Source: CAD feature listing. Evaluate the final solid. Frame: model axes, mm. Give positions to 0.01 mm unless a question says otherwise; leave off trailing zeros. Write each loop counter-clockwise with the first axis right and the second up, starting at its lowest first coordinate (ties: lowest second). Pieces come first, ordered by that corner, then holes. Notation, with made-up numbers: (80, -30.75) -> (99, -30.75) arc R23 cw to (99, 1.25) -> close; hole circle Ø3 at (-24, 59.5). An arc over 180 degrees is marked (long way). Use one line per item in the form item = value. Start each with the question number.
(1) Cut plane B-B, the plane y = 1.9. Output: boundary loops of the cut face in (x, z).
(2) Cut plane C-C, the plane x = -4. Output: boundary loops of the cut face in (y, z), and give its area (3 significant figures).
(3) Cut plane D-D, the plane y = -1.8. Output: boundary loops of the cut face in (x, z), and give its area (3 significant figures).
(4) Cut plane A-A, the plane z = 15. Output: boundary loops of the cut face in (x, y), and give its area (3 significant figures).
(5) Material intervals for line 1 along Z through (x, y) = (-0.5, -2.15); line 2 along Z through (x, y) = (3.5, -1.65); line 3 along X through (y, z) = (2.3, -13.5), sorted ascending. Write a range as from..to.
from build123d import *

# Parameters (mm, degrees)
BOSS_EXTRUDE1_DEPTH = 17.5
CUT_EXTRUDE1_START  = -2.5
CUT_EXTRUDE1_DEPTH  = 5


# Read off the part's stored shape, not the designer's step: Cut-Extrude1
with BuildPart() as part:
    # Sketch1 → Boss-Extrude1 (new, symmetric)
    with BuildSketch(Plane.XY):
        with BuildLine():
            Line((-3.5, -2.5), (3.5, -2.5))
            ThreePointArc((3.5, -2.5), (4.560660172, -2.060660172), (5, -1))
            Line((5, -1), (5, 1))
            ThreePointArc((5, 1), (4.560660172, 2.060660172), (3.5, 2.5))
            Line((3.5, 2.5), (-3.5, 2.5))
            ThreePointArc((-3.5, 2.5), (-4.560660172, 2.060660172), (-5, 1))
            Line((-5, 1), (-5, -1))
            ThreePointArc((-5, -1), (-4.560660172, -2.060660172), (-3.5, -2.5))
        make_face()
    extrude(amount=BOSS_EXTRUDE1_DEPTH, both=True)

    # Cut-Extrude1 outline → Cut-Extrude1 (cut)
    with BuildSketch(Plane(origin=(0, 0, 0), x_dir=(1, 0, 0), z_dir=(0, 1, 0)).offset(CUT_EXTRUDE1_START)):
        with BuildLine():
            ThreePointArc((-1.03e-07, -17.5), (-2.52646852, -17.316667024), (-5.000001513, -16.77050938))
            Line((-5.000001513, -16.77050938), (-5, -17.5))
            Line((-5, -17.5), (-1.03e-07, -17.5))
        make_face()
        with BuildLine():
            ThreePointArc((5.000001513, -16.77050938), (2.526468418, -17.316667039), (-1.03e-07, -17.5))
            Line((-1.03e-07, -17.5), (5, -17.5))
            Line((5, -17.5), (5.000001513, -16.77050938))
        make_face()
        with BuildLine():
            Line((-5, 17.5), (-5.000001513, 16.77050938))
            ThreePointArc((-5.000001513, 16.77050938), (-2.526468418, 17.316667039), (1.03e-07, 17.5))
            Line((1.03e-07, 17.5), (-5, 17.5))
        make_face()
        with BuildLine():
            Line((5, 17.5), (1.03e-07, 17.5))
            ThreePointArc((1.03e-07, 17.5), (2.52646852, 17.316667024), (5.000001513, 16.77050938))
            Line((5.000001513, 16.77050938), (5, 17.5))
        make_face()
    extrude(amount=CUT_EXTRUDE1_DEPTH, mode=Mode.SUBTRACT)


solid = part.part
Geometry says:
q1.outline = (-4.7, -16.86) arc R17.5 ccw to (4.7, -16.86) -> (4.7, 16.86) arc R17.5 ccw to (-4.7, 16.86) -> close
q2.outline = (-2.41, -17.04) -> (2.41, -17.04) -> (2.41, 17.04) -> (-2.41, 17.04) -> close
q2.area = 165 mm^2
q3.outline = (-4.77, -16.84) arc R17.5 ccw to (4.77, -16.84) -> (4.77, 16.84) arc R17.5 ccw to (-4.77, 16.84) -> close
q3.area = 330 mm^2
q4.outline = (-5, -1) arc R1.5 ccw to (-3.5, -2.5) -> (3.5, -2.5) arc R1.5 ccw to (5, -1) -> (5, 1) arc R1.5 ccw to (3.5, 2.5) -> (-3.5, 2.5) arc R1.5 ccw to (-5, 1) -> close
q4.area = 48.1 mm^2
q5.line_1 = -17.49..17.49
q5.line_2 = -17.15..17.15
q5.line_3 = -4.25..4.25
